Could you check a few things on this model? Use its own coordinates, in mm. Give positions to 0.01 mm unless a question says otherwise; leave off trailing zeros. Loops run counter-clockwise (first coordinate to the right, second up) from the corner with the lowest first, then second, coordinate; pieces in that order, holes last. Notation, with made-up numbers: (-4.75, 45) - (16.25, 45) arc R25 cw to (16.25, 76) - close; hole circle Ø11 at (44, 32). An arc over 180 degrees is marked (long way). Write each question's results on one line, items separated by ' | '. Start each with the question number.
(1) For pin 1 (6 mm diameter, centred on x = 17.5, z = 1171, fed in from -Y), with a flat end and sliding along its axis, tell me the tip position at first contact or that it passes through.
(2) Suppose I cut it at A-A (y = 13.25). Please give me the cut outline in (x, z).
(3) Suppose I cut it at B-B (x = 41.5). Please give me the cut outline in (y, z).
(4) Suppose I cut it at C-C (z = 1024). Please give me the cut outline in (x, y), and give its area (3 significant figures).
(5) I need wall thicknesses on line 1 (X direction, y = 7.25, z = 1576); line 2 (Y direction, x = 8, z = 1288). Which ranges of each line are inside material? Lowest first, please.
Autodesk Inventor part; units mm, degrees
ref_plane "YZ Plane" through (0, 0, 0) normal (1, 0, 0) x (0, 1, 0)
ref_plane "XZ Plane" through (0, 0, 0) normal (0, 1, 0) x (-1, 0, 0)
ref_plane "XY Plane" through (0, 0, 0) normal (0, 0, 1) x (1, 0, 0)
sketch "Sketch1" plane through (0, 0, 0) normal (0, 0, 1) x (1, 0, 0)
  line L0 (0, 0) -> (50.8, 0)
  line L1 (50.8, 0) -> (50.8, 25.4)
  line L2 (50.8, 25.4) -> (0, 25.4)
  line L3 (0, 25.4) -> (0, 0)
  dimension "d0" = 50.8
  dimension "d1" = 25.4
extrude "Extrusion1" add sketch "Sketch1" along normal blind 1828.8
shell "Shell1" thickness 1.5875 removed faces 2 at (16.9333, 8.4667, 0) at (16.9333, 8.4667, 1828.8)
equation "\"d2\" = Length"
equation "\"Length\" = 1828.8"
properties part number "Box Tube"
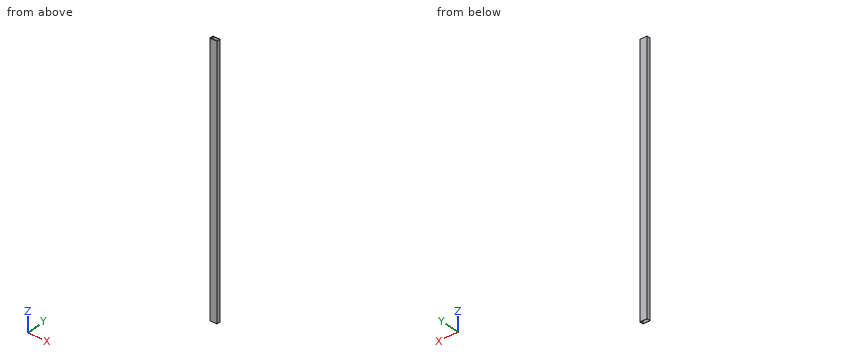
Output values:
1) pin 1: y = 0
2) outline: (0, 0) - (1.59, 0) - (1.59, 1828.8) - (0, 1828.8) - close; (49.21, 0) - (50.8, 0) - (50.8, 1828.8) - (49.21, 1828.8) - close
3) outline: (0, 0) - (1.59, 0) - (1.59, 1828.8) - (0, 1828.8) - close; (23.81, 0) - (25.4, 0) - (25.4, 1828.8) - (23.81, 1828.8) - close
4) outline: (0, 0) - (50.8, 0) - (50.8, 25.4) - (0, 25.4) - close; hole (1.59, 1.59) - (49.21, 1.59) - (49.21, 23.81) - (1.59, 23.81) - close | area: 232 mm2
5) line 1: 0 to 1.59, 49.21 to 50.8 | line 2: 0 to 1.59, 23.81 to 25.4
